from build123d import *

# Parameters (mm, degrees)
SKETCH_1_W          = 43
SKETCH_1_H          = 170
EXTRUDE_1_DEPTH     = 16
SKETCH_3_W          = 39
SKETCH_3_H          = 152
CUT_EXTRUDE_1_DEPTH = 177.08236709
FILLET_3_R          = 8


with BuildPart() as part:
    # Эскиз1 → Бобышка-Вытянуть1 (new body)
    with BuildSketch(Plane.XY):
        with Locations((21.5, 85)):
            Rectangle(SKETCH_1_W, SKETCH_1_H)
    extrude(amount=EXTRUDE_1_DEPTH)

    # Эскиз3 → Вырез-Вытянуть1 (cut, through all)
    with BuildSketch(Plane.XY.offset(16)):
        with Locations((21.5, 85)):
            Rectangle(SKETCH_3_W, SKETCH_3_H)
    extrude(amount=-CUT_EXTRUDE_1_DEPTH, mode=Mode.SUBTRACT)

    # Скругление3
    fillet_3_edges = [part.edges().sort_by_distance(p)[0] for p in [
        (43, 0, 8),
        (0, 0, 8),
    ]]
    fillet(fillet_3_edges, radius=FILLET_3_R)


solid = part.part
Source: CAD feature listing. Evaluate the final solid. Frame: model axes, mm. A direction names the side the tool comes from. Round coordinates to 2 decimals unless told otherwise and drop trailing zeros. Loops run counter-clockwise (first coordinate to the right, second up) from the corner with the lowest first, then second, coordinate; pieces in that order, holes last. Notation, with made-up numbers: M 63.25,28.5 L 102.25,28.5 A18 ccw 102.25,34.5 Z; hole C 32,-34 d9. An arc over 180 degrees is marked long. Return JSON: item names as keys, results as strings. Group by question number.
1. Pin query (flat end, axial travel): pin 1 (4 mm diameter, centred on x = 38.5, z = 2.5, fed in from -Y). Return the tip coordinate at first contact, or that it passes through.
2. Material intervals for line 1 along X through (y, z) = (73.5, 12.25); line 2 along Y through (x, z) = (35.5, 1); line 3 along Y through (x, z) = (36, 9.5), sorted ascending. Write a range as from..to.
3. Section query B-B on y = 157. Output: boundary loops of the cut face in (x, z), and give its area (3 significant figures).
4. Section query A-A on x = 27. Output: boundary loops of the cut face in (y, z).
5. Reachability of faces 1 (the face through (1, 85, 0)), 2 (the face through (21, 161, 8)) from +Z, -Z, +X, -X, +Y, -Y: full face, straight path, thin tool, end or side. Return the list, or none.
6. Mould query, pull axis X, two halves, no side actions, for faces 3 (the face through (1, 85, 16)), 4 (the face through (40.594, 2.281, 8.112)), 5 (the face through (2, 84, 8)). Classes: released by +X, released by -X, zero draft, split by the parting line, or undercut.
7. Section query C-C on z = 2. Output: boundary loops of the cut face in (x, y), and give its area (3 significant figures).
Checks:
{
 "1": {"pin 1": "stops at y = 0.14"},
 "2": {"line 1": "x = 0..2, 41..43", "line 2": "y = 0.02..9, 161..170", "line 3": "y = 0.06..9, 161..170"},
 "3": {"outline": "M 0,0 L 2,0 L 2,16 L 0,16 Z; M 41,0 L 43,0 L 43,16 L 41,16 Z", "area": "64.0 mm²"},
 "4": {"outline": "M 0,0 L 9,0 L 9,16 L 0,16 Z; M 161,0 L 170,0 L 170,16 L 161,16 Z"},
 "5": {"face 1": "-Z, +X, -X, +Y, -Y", "face 2": "+Z, -Z"},
 "6": {"face 3": "zero draft", "face 4": "released by +X", "face 5": "undercut"},
 "7": {"outline": "M 0,8 A8 ccw 8,0 L 35,0 A8 ccw 43,8 L 43,170 L 0,170 Z; hole M 2,9 L 41,9 L 41,161 L 2,161 Z", "area": "1,350 mm²"}
}
